Can you work these out from the model? Positions are in its coordinate system, mm. A direction names the side the tool comes from. Give positions to 0.01 mm unless a question says otherwise; leave off trailing zeros. Order: outer loops, then holes, each group sorted by start corner. A loop starts at its lowest first (then second) coordinate and runs counter-clockwise, first axis right, second up. Notation, with made-up numbers: M 63,2.25 L 92,2.25 A11 ccw 92,16.25 Z; hole C -4.75,66.5 d10. An arc over 180 degrees is marked long. One line per question, with ' | ' between items. Start each with the question number.
1) Please list where these lines run through material, in increasing order: line 1 along Y through (x, z) = (-991, 6.5); line 2 along Y through (x, z) = (-936.5, 8.5); line 3 along X through (y, z) = (590.5, 13). Write a range as [from, to].
2) Thinking about a two-plate mould opening in X: for faces 4 (the flat face through (-999.102, 598, 9)), 5 (the flat face through (-961.002, 379, 9)), 6 (the flat face through (-1196, 344.389, 9)), which applies, +X half, -X half, draft (parallel to the pull), parting line (faces both ways), or undercut?
3) If we section it at A-A, the plane z = 9.5: Please give me the cut outline in (x, y), plus the area to 3 significant figures.
4) For faces 1 (the flat face through (-1196, 602, 18.542)), 2 (the flat face through (-1000, 808.447, 9)), 3 (the flat face through (-868, 630.139, 9)), which set-ups out of +Z, -Z, +X, -X, +Y, -Y let a thin tool reach every point of the face, with its end or its side?
```python
from build123d import *

# Parameters (mm, degrees)
F0_W     = 76.2
F0_H     = 18.542
F0_R     = 30.48
F1_DEPTH = 18.542
F2_DEPTH = 18.542


with BuildPart() as f1:
    # F0 (on Top) → F1 (new body)
    with BuildSketch(Plane.XY):
        Polygon((-732.4015087128, 852.3886724055), (-1646.8015087128, 852.3886724055), (-1646.8015087128, 547.5886724055), (-1646.8015087128, 344.3886724055), (-732.4015087128, 344.3886724055), (-732.4015087128, 369.7886724055), (-732.4015087128, 566.6386724055), (-999.1015087128, 566.6386724055), (-999.1015087128, 630.1386724055), (-732.4015087128, 630.1386724055), (-732.4015087128, 808.4466724055), (-732.4015087128, 826.9886724055), align=None)
        with Locations((-999.1015087128, 379.0596724055)):
            Rectangle(F0_W, F0_H, mode=Mode.SUBTRACT)
        with Locations((-846.7015087128, 379.0596724055)):
            Rectangle(F0_W, F0_H, mode=Mode.SUBTRACT)
        with Locations((-1356.4279079437, 598.3886724055)):
            Circle(F0_R, mode=Mode.SUBTRACT)
        with Locations((-999.1015087128, 817.7176724055)):
            Rectangle(F0_W, F0_H, mode=Mode.SUBTRACT)
        with Locations((-846.7015087128, 817.7176724055)):
            Rectangle(F0_W, F0_H, mode=Mode.SUBTRACT)
    extrude(amount=F1_DEPTH)

    # F0 (on Top) → F2 (join)
    with BuildSketch(Plane.XY):
        Polygon((-732.4015087128, 852.3886724055), (-1646.8015087128, 852.3886724055), (-1646.8015087128, 547.5886724055), (-1646.8015087128, 344.3886724055), (-732.4015087128, 344.3886724055), (-732.4015087128, 369.7886724055), (-732.4015087128, 566.6386724055), (-999.1015087128, 566.6386724055), (-999.1015087128, 630.1386724055), (-732.4015087128, 630.1386724055), (-732.4015087128, 808.4466724055), (-732.4015087128, 826.9886724055), align=None)
        with Locations((-999.1015087128, 379.0596724055)):
            Rectangle(F0_W, F0_H, mode=Mode.SUBTRACT)
        with Locations((-846.7015087128, 379.0596724055)):
            Rectangle(F0_W, F0_H, mode=Mode.SUBTRACT)
        with Locations((-1356.4279079437, 598.3886724055)):
            Circle(F0_R, mode=Mode.SUBTRACT)
        with Locations((-999.1015087128, 817.7176724055)):
            Rectangle(F0_W, F0_H, mode=Mode.SUBTRACT)
        with Locations((-846.7015087128, 817.7176724055)):
            Rectangle(F0_W, F0_H, mode=Mode.SUBTRACT)
    extrude(amount=F2_DEPTH)


solid = f1.part
```
Results found:
1) line 1: y = [344.39, 369.79], [388.33, 566.64], [630.14, 808.45], [826.99, 852.39] | line 2: y = [344.39, 566.64], [630.14, 852.39] | line 3: x = [-1646.8, -1385.87], [-1326.99, -999.1]
2) face 4: +X half | face 5: undercut | face 6: draft
3) outline: M -1646.8,344.39 L -732.4,344.39 L -732.4,566.64 L -999.1,566.64 L -999.1,630.14 L -732.4,630.14 L -732.4,852.39 L -1646.8,852.39 Z; hole C -1356.43,598.39 d60.96; hole M -1037.2,369.79 L -961,369.79 L -961,388.33 L -1037.2,388.33 Z; hole M -1037.2,808.45 L -961,808.45 L -961,826.99 L -1037.2,826.99 Z; hole M -884.8,369.79 L -808.6,369.79 L -808.6,388.33 L -884.8,388.33 Z; hole M -884.8,808.45 L -808.6,808.45 L -808.6,826.99 L -884.8,826.99 Z | area: 439,000 mm²
4) face 1: +Z, +X, -X, +Y, -Y | face 2: +Z, -Z | face 3: +Z, -Z, +X
